```python
from build123d import *
from build123d.topology import SkipClean

# Parameters (mm, degrees)
SKETCH_1_R          = 44
SKETCH_1_R_2        = 11.25
SKETCH_1_R_3        = 2.1
EXTRUDE_1_DEPTH     = 4
SKETCH_2_OUTSIDE_W  = 114.904
SKETCH_2_OUTSIDE_H  = 114.904
SKETCH_2_OUTSIDE_R  = 24.625
CUT_EXTRUDE_1_DEPTH = 10


with BuildPart() as part:
    # 草图1 → 凸台-拉伸1 (new body)
    with BuildSketch(Plane.XY):
        Circle(SKETCH_1_R)
        Circle(SKETCH_1_R_2, mode=Mode.SUBTRACT)
        with Locations((0, 17.25)):
            Circle(SKETCH_1_R_3, mode=Mode.SUBTRACT)
        with Locations((14.938938215, 8.625)):
            Circle(SKETCH_1_R_3, mode=Mode.SUBTRACT)
        with Locations((14.938938215, -8.625)):
            Circle(SKETCH_1_R_3, mode=Mode.SUBTRACT)
        with Locations((0, -17.25)):
            Circle(SKETCH_1_R_3, mode=Mode.SUBTRACT)
        with Locations((-14.938938215, -8.625)):
            Circle(SKETCH_1_R_3, mode=Mode.SUBTRACT)
        with Locations((-14.938938215, 8.625)):
            Circle(SKETCH_1_R_3, mode=Mode.SUBTRACT)
        with BuildLine():
            ThreePointArc((23.542096205, 28.056377729), (0, 36.625), (-23.542096205, 28.056377729))
            ThreePointArc((-23.542096205, 28.056377729), (-24.281637205, 19.603385412), (-15.828644889, 18.863844412))
            ThreePointArc((-15.828644889, 18.863844412), (0, 24.625), (15.828644889, 18.863844412))
            ThreePointArc((15.828644889, 18.863844412), (24.281637205, 19.603385412), (23.542096205, 28.056377729))
        make_face(mode=Mode.SUBTRACT)
        with BuildLine():
            ThreePointArc((12.526487749, -34.416242236), (31.718180414, -18.3125), (36.068583954, 6.359864507))
            ThreePointArc((36.068583954, 6.359864507), (29.11784837, 11.226821959), (24.250890918, 4.276086375))
            ThreePointArc((24.250890918, 4.276086375), (21.325875568, -12.3125), (8.422246029, -23.139930787))
            ThreePointArc((8.422246029, -23.139930787), (4.836211165, -30.830207372), (12.526487749, -34.416242236))
        make_face(mode=Mode.SUBTRACT)
        with BuildLine():
            ThreePointArc((-36.068583954, 6.359864507), (-31.718180414, -18.3125), (-12.526487749, -34.416242236))
            ThreePointArc((-12.526487749, -34.416242236), (-4.836211165, -30.830207372), (-8.422246029, -23.139930787))
            ThreePointArc((-8.422246029, -23.139930787), (-21.325875568, -12.3125), (-24.250890918, 4.276086375))
            ThreePointArc((-24.250890918, 4.276086375), (-29.11784837, 11.226821959), (-36.068583954, 6.359864507))
        make_face(mode=Mode.SUBTRACT)
    extrude(amount=EXTRUDE_1_DEPTH)

    # 草图2 outside → 切除-拉伸1 (cut)
    with SkipClean():  # the faces are left unmerged after this step: merging them gives an invalid solid
        with BuildSketch(Plane.XY.offset(4)):
            Rectangle(SKETCH_2_OUTSIDE_W, SKETCH_2_OUTSIDE_H)
            Circle(SKETCH_2_OUTSIDE_R, mode=Mode.SUBTRACT)
        extrude(amount=-CUT_EXTRUDE_1_DEPTH, mode=Mode.SUBTRACT)


solid = part.part
```
Geometry: final body of the model. Coordinates: model frame, mm. Coordinates: 2 decimals unless noted, no trailing zeros. Write each loop counter-clockwise with the first axis right and the second up, starting at its lowest first coordinate (ties: lowest second). Pieces come first, ordered by that corner, then holes. Notation, with made-up numbers: M 50.5,63 L 93.5,63 A18 ccw 93.5,97 Z; hole C 81.5,28 d11. An arc over 180 degrees is marked long. Use CSV: the item, a comma, the result in double quotes. Start each with the question number.
1. Mould query, pull axis Y, two halves, no side actions, for faces 1 (the face through (14.666, -6.543, 1.972)), 2 (the face through (-0.273, -15.168, 1.972)), 3 (the face through (11, -5, 0)). Classes: pulls with the +Y half, pulls with the -Y half, needs draft (parallel to the pull), parting line crosses it, or undercut.
2. First-contact query: P1, Ø2, axis at y = -8.5, z = 1.5, coming from the +X side; P2, Ø4, axis at x = 14.94, y = -8.62, coming from the -Z side; P3, Ø1.5, axis at x = -16, z = 2, coming from the -Y side. Flat tips, straight axial feed; report the tip coordinate or a pass-through.
3. Cut plane B-B on y = -3. Return the cut outline in (x, z).
4. Cut plane D-D on y = -17.25. Return the cut outline in (x, z), plus the area to 3 significant figures.
5. Cut plane A-A on x = 0. Return the cut outline in (y, z) (3 decimals), plus the area to 3 significant figures.
6. Cut plane C-C on z = 3. Return the cut outline in (x, y) (3 decimals).
7. Ray query, probe 1 along Y at (x, z) = (0, 0.95) (3 decimals); probe 2 along X at (y, z) = (7.5, 0.6); probe 3 along Y at (x, z) = (15.5, 3.2). Return the intervals inside material, ascending.
Entries:
1,face 1,"undercut"
1,face 2,"undercut"
1,face 3,"needs draft"
2,P1,"x = 23.46"
2,P2,"through"
2,P3,"y = -19.33"
3,outline,"M -24.44,0 L -10.84,0 L -10.84,4 L -24.44,4 Z; M 10.84,0 L 24.44,0 L 24.44,4 L 10.84,4 Z"
4,outline,"M -17.57,0 L -2.1,0 L -2.1,4 L -17.57,4 Z; M 2.1,0 L 17.57,0 L 17.57,4 L 2.1,4 Z"
4,area,"124 mm²"
5,outline,"M -24.625,0 L -19.35,0 L -19.35,4 L -24.625,4 Z; M -15.15,0 L -11.25,0 L -11.25,4 L -15.15,4 Z; M 11.25,0 L 15.15,0 L 15.15,4 L 11.25,4 Z; M 19.35,0 L 24.625,0 L 24.625,4 L 19.35,4 Z"
5,area,"73.4 mm²"
6,outline,"C 0,0 d49.25; hole C -14.939,-8.625 d4.2; hole C -14.939,8.625 d4.2; hole C 0,0 d22.5; hole C 0,-17.25 d4.2; hole C 0,17.25 d4.2; hole C 14.939,-8.625 d4.2; hole C 14.939,8.625 d4.2"
7,probe 1,"-24.625 to -19.35, -15.15 to -11.25, 11.25 to 15.15, 19.35 to 24.625"
7,probe 2,"-23.46 to -16.71, -13.17 to -8.39, 8.39 to 13.17, 16.71 to 23.46"
7,probe 3,"-19.13 to -10.65, -6.6 to 6.6, 10.65 to 19.13"
